Autodesk Inventor part; units mm, degrees
ref_plane "YZ Plane" through (0, 0, 0) normal (1, 0, 0) x (0, 1, 0)
ref_plane "XZ Plane" through (0, 0, 0) normal (0, 1, 0) x (-1, 0, 0)
ref_plane "XY Plane" through (0, 0, 0) normal (0, 0, 1) x (1, 0, 0)
sketch "Boceto1" plane through (0, 0, 0) normal (0, 1, 0) x (-1, 0, 0)
  line L0 (39.25, 31.5) -> (-39.25, 31.5)
  line L1 (-39.25, 31.5) -> (-39.25, -31.5)
  line L2 (-39.25, -31.5) -> (39.25, -31.5)
  line L3 (39.25, -31.5) -> (39.25, 31.5)
  line L4 (39.25, 31.5) -> (-39.25, -31.5) construction
  line L5 (-39.25, 31.5) -> (39.25, -31.5) construction
  point P0 (0, 0)
  dimension "d0" = 78.5
  dimension "d1" = 63
extrude "Extrusión1" add sketch "Boceto1" along normal blind 5
sketch "Boceto2" plane through (0, 5, 0) normal (0, 1, 0) x (1, 0, 0)
  circle A0 centre (31, -23.25) radius 7.25
  line L0 (0, 0) -> (0, -1.7079)
  line L1 (-39.25, -31.5) -> (39.25, -31.5)
  line L2 (0, 0) -> (-6.7024, 0)
  line L3 (31, -30.5) -> (-1.6149, -30.5)
  line L4 (38.25, -23.25) -> (38.25, -18.8527)
  line L5 (39.25, -31.5) -> (39.25, 31.5)
  line L6 (31, -23.25) -> (31, -17.7026)
  line L7 (31, -16) -> (21.1009, -16)
  line L8 (31, -0.5) -> (21.1009, -0.5)
  circle A1 centre (31, -7.75) radius 7.25
  line L9 (31, -15) -> (-1.6149, -15)
  line L10 (31, 15) -> (21.1009, 15)
  circle A2 centre (31, 7.75) radius 7.25
  line L11 (31, 0.5) -> (-1.6149, 0.5)
  line L12 (31, 30.5) -> (21.1009, 30.5)
  circle A3 centre (31, 23.25) radius 7.25
  line L13 (31, 16) -> (-1.6149, 16)
  line L14 (39.25, 31.5) -> (-39.25, 31.5)
  circle A4 centre (15.5, -23.25) radius 7.25
  circle A5 centre (15.5, -7.75) radius 7.25
  circle A6 centre (15.5, 7.75) radius 7.25
  circle A7 centre (15.5, 23.25) radius 7.25
  circle A8 centre (0, -23.25) radius 7.25
  circle A9 centre (0, -7.75) radius 7.25
  circle A10 centre (0, 7.75) radius 7.25
  circle A11 centre (0, 23.25) radius 7.25
  circle A12 centre (-15.5, -23.25) radius 7.25
  circle A13 centre (-15.5, -7.75) radius 7.25
  circle A14 centre (-15.5, 7.75) radius 7.25
  circle A15 centre (-15.5, 23.25) radius 7.25
  circle A16 centre (-31, -23.25) radius 7.25
  circle A17 centre (-31, -7.75) radius 7.25
  circle A18 centre (-31, 7.75) radius 7.25
  circle A19 centre (-31, 23.25) radius 7.25
  line L15 (22.75, -23.25) -> (22.75, -18.6411)
  line L16 (23.75, -23.25) -> (23.75, -18.1365)
  line L17 (-38.25, -23.25) -> (-38.25, -18.441)
  line L18 (-39.25, 31.5) -> (-39.25, -31.5)
  point P0 (-1.5837, 0)
  point P1 (38.25, -7.75)
  point P2 (38.25, 7.75)
  point P3 (38.25, 23.25)
  point P4 (15.5, -30.5)
  point P5 (15.5, -16)
  point P6 (15.5, -15)
  point P7 (22.75, -7.75)
  point P8 (15.5, -0.5)
  point P9 (15.5, 0.5)
  point P10 (22.75, 7.75)
  point P11 (15.5, 15)
  point P12 (15.5, 16)
  point P13 (22.75, 23.25)
  point P14 (15.5, 30.5)
  point P15 (0, -30.5)
  point P16 (7.25, -23.25)
  point P17 (0, -16)
  point P18 (0, -15)
  point P19 (7.25, -7.75)
  point P20 (0, -0.5)
  point P21 (0, 0.5)
  point P22 (7.25, 7.75)
  point P23 (0, 15)
  point P24 (0, 16)
  point P25 (7.25, 23.25)
  point P26 (0, 30.5)
  point P27 (-15.5, -30.5)
  point P28 (-8.25, -23.25)
  point P29 (-15.5, -16)
  point P30 (-15.5, -15)
  point P31 (-8.25, -7.75)
  point P32 (-15.5, -0.5)
  point P33 (-15.5, 0.5)
  point P34 (-8.25, 7.75)
  point P35 (-15.5, 15)
  point P36 (-15.5, 16)
  point P37 (-8.25, 23.25)
  point P38 (-15.5, 30.5)
  point P39 (-31, -30.5)
  point P40 (-23.75, -23.25)
  point P41 (-31, -16)
  point P42 (-31, -15)
  point P43 (-23.75, -7.75)
  point P44 (-31, -0.5)
  point P45 (-31, 0.5)
  point P46 (-23.75, 7.75)
  point P47 (-31, 15)
  point P48 (-31, 16)
  point P49 (-23.75, 23.25)
  point P50 (-31, 30.5)
  dimension "d4" = 14.5
  dimension "d6" = 23.25
  dimension "d13" = 7.25
  dimension "d14" = 1
  dimension "d15" = 7.25
  dimension "d16" = 1
  dimension "d19" = 15.5
  dimension "d24" = 1
  dimension "d25" = 1
  dimension "d28" = 15.5
  dimension "d33" = 1
  dimension "d34" = 1
extrude "Extrusión2" cut sketch "Boceto2" against normal blind 3.5 contours A0 | A8 | A4 | A1 | A9 | A5 | A2 | A10 | A6 | A3 | A11 | A7 | A12 | A13 | A14 | A15 | A16 | A17 | A18 | A19
sketch "Boceto3" plane through (31, 1.5, 23.25) normal (0, 1, 0) x (1, 0, 0)
  circle A0 centre (0, 0) radius 5
  line L0 (0, 0) -> (0, 5.1334)
  circle A1 centre (0, 15.5) radius 5
  circle A2 centre (0, 31) radius 5
  circle A3 centre (0, 46.5) radius 5
  circle A4 centre (0, 15.5) radius 7.25
  line L1 (0, 0) -> (-4.4758, 0)
  circle A5 centre (-15.5, 46.5) radius 5
  circle A6 centre (-15.5, 31) radius 5
  circle A7 centre (-15.5, 15.5) radius 5
  circle A8 centre (-15.5, 0) radius 5
  circle A9 centre (-31, 46.5) radius 5
  circle A10 centre (-31, 31) radius 5
  circle A11 centre (-31, 15.5) radius 5
  circle A12 centre (-31, 0) radius 5
  circle A13 centre (-46.5, 46.5) radius 5
  circle A14 centre (-46.5, 31) radius 5
  circle A15 centre (-46.5, 15.5) radius 5
  circle A16 centre (-46.5, 0) radius 5
  circle A17 centre (-62, 46.5) radius 5
  circle A18 centre (-62, 31) radius 5
  circle A19 centre (-62, 15.5) radius 5
  circle A20 centre (-62, 0) radius 5
  circle A21 centre (-15.5, 0) radius 7.25
  circle A22 centre (0, 0) radius 7.25
  point P0 (-31, 23.25)
  dimension "d10" = 10
  dimension "d37" = 15.5
  dimension "d44" = 15.5
  dimension "d49" = 2.25
extrude "Extrusión3" cut sketch "Boceto3" against normal blind 4 contours A0 | A1 | A2 | A3 | A5 | A6 | A7 | A8 | A9 | A10 | A11 | A12 | A13 | A14 | A15 | A16 | A17 | A18 | A19 | A20
properties part number "battery_pack_base"
Model file for the job. Use its own axes, mm. A direction names the side the tool comes from. Give positions to 0.01 mm unless a question says otherwise; leave off trailing zeros. Use CSV: the item, a comma, the result in double quotes. Start each with the question number.
1) Slice it at A-A on y = 2.45. Give the number of separate pieces and of enclosed holes in the cut face, plus the area to 3 significant figures.
2) Mould opens along X. For faces 1 (the cylindrical face through (-1.08, 0.76, -18.37)), 2 (the flat face through (-39.25, 2, 0)), 3 (the flat face through (1, 2, -31.5)) say: released by +X, released by -X, zero draft, split by the parting line, or undercut.
3) Tool access for faces 4 (the cylindrical face through (-16.58, 0.76, -18.37)), 5 (the cylindrical face through (-38.243, 3.274, 22.931)): list every direction of +Z, -Z, +X, -X, +Y, -Y with a clear straight run to the whole face (end or side of a thin tool).
4) Wall check: line 1 (Z direction, x = -31, y = 0.5); line 2 (X direction, y = 1.6, z = -18); line 3 (X direction, y = 2.65, z = 7.75). Give the ranges that are in metal, low to high.
5) Flat gauge pins, fed straight in: pin 1 Ø11.5 at (x, z) = (-31, -7.75) entering from +Y; pin 2 Ø8 at (x, z) = (31, 7.75) entering from +Y. Where does each tip first touch, or does it go through?
Computed values:
1,separate pieces,"1"
1,enclosed holes,"20"
1,area,"1,640 mm^2"
2,face 1,"undercut"
2,face 2,"released by -X"
2,face 3,"zero draft"
3,face 4,"+Y, -Y"
3,face 5,"+Y"
4,line 1,"z = -31.5 to -28.25, -18.25 to -12.75, -2.75 to 2.75, 12.75 to 18.25, 28.25 to 31.5"
4,line 2,"x = -39.25 to -36, -26 to -20.5, -10.5 to -5, 5 to 10.5, 20.5 to 26, 36 to 39.25"
4,line 3,"x = -39.25 to -38.25, -23.75 to -22.75, -8.25 to -7.25, 7.25 to 8.25, 22.75 to 23.75, 38.25 to 39.25"
5,pin 1,"stops at y = 1.5"
5,pin 2,"passes through"
